Geometry: see drawing. Coordinates: mm, zero at the bounding-box minimum. A direction names the side the tool comes from. Coordinates: 2 decimals unless noted, no trailing zeros. Order: outer loops, then holes, each group sorted by start corner. A loop starts at its lowest first (then second) coordinate and runs counter-clockwise, first axis right, second up. Notation, with made-up numbers: M 38,39 L 75,39 A23 ccw 75,61 Z; hole C -16,-21.5 d11. An arc over 180 degrees is marked long. Answer in a Markdown table with one row per item.
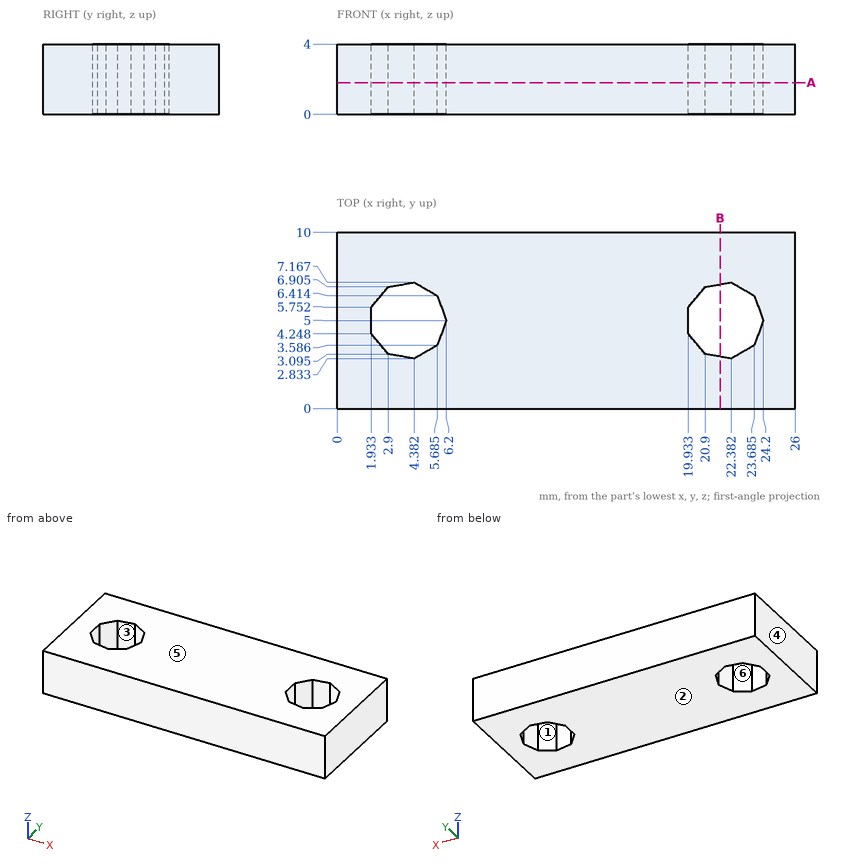
1) Cut plane A-A, the plane z = 1.8. Output: boundary loops of the cut face in (x, y) (1 decimal), and give its area (3 significant figures).
Resolved:
| item | result |
|---|---|
| outline | M 0,0 L 26,0 L 26,10 L 0,10 Z; hole M 1.9,4.2 L 2.9,3.1 L 4.4,2.8 L 5.7,3.6 L 6.2,5 L 5.7,6.4 L 4.4,7.2 L 2.9,6.9 L 1.9,5.8 Z; hole M 19.9,4.2 L 20.9,3.1 L 22.4,2.8 L 23.7,3.6 L 24.2,5 L 23.7,6.4 L 22.4,7.2 L 20.9,6.9 L 19.9,5.8 Z |
| area | 232 mm2 |
2) Reachability of the marked faces 1 and 2 from +Z, -Z, +X, -X, +Y, -Y: full face, straight path, thin tool, end or side. Return the list, or none.
Resolved:
| item | result |
|---|---|
| face 1 | +Z, -Z |
| face 2 | -Z, +X, -X, +Y, -Y |
3) Cut plane B-B, the plane x = 21.75. Output: boundary loops of the cut face in (y, z) (1 decimal).
Resolved:
| item | result |
|---|---|
| outline | M 0,0 L 2.9,0 L 2.9,4 L 0,4 Z; M 7.1,0 L 10,0 L 10,4 L 7.1,4 Z |
4) Contact query for a flat-ended pin moving along its axis: pin 1 (1.5 mm diameter, centred on x = 6.5, y = 9, fed in from -Z). Output: stop coordinate, or through.
Resolved:
| item | result |
|---|---|
| pin 1 | stops at z = 0 |
5) Mould query, pull axis X, two halves, no side actions, for the marked faces 3, 4, 5 and 6. Classes: +X half, -X half, draft (parallel to the pull), parting line (faces both ways), or undercut.
Resolved:
| item | result |
|---|---|
| face 3 | undercut |
| face 4 | -X half |
| face 5 | draft |
| face 6 | undercut |
6) Material intervals for probe 1 along X at (y, z) = (3.5, 3) (1 decimal); probe 2 along X at (y, z) = (6, 0.8) (1 decimal); probe 3 along Y at (x, z) = (3, 1.6), sorted ascending.
Resolved:
| item | result |
|---|---|
| probe 1 | x = 0 to 2.6, 5.5 to 20.6, 23.5 to 26 |
| probe 2 | x = 0 to 2.1, 5.8 to 20.1, 23.8 to 26 |
| probe 3 | y = 0 to 3.08, 6.92 to 10 |
